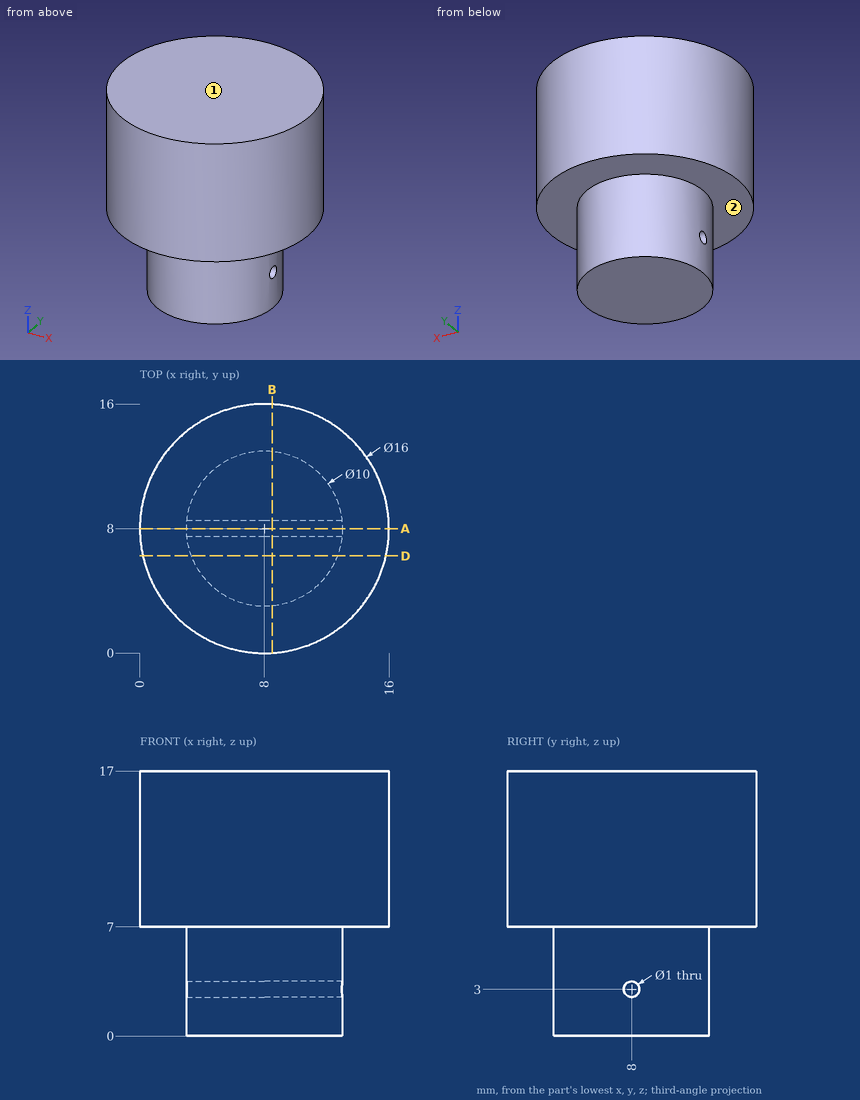
The figure shows three views and two pictorial views of one solid part (mm, origin at its lowest corner). Answer the questions. A direction names the side the tool comes from. Round coordinates to 2 decimals unless told otherwise and drop trailing zeros. Write each loop counter-clockwise with the first axis right and the second up, starting at its lowest first coordinate (ties: lowest second). Pieces come first, ordered by that corner, then holes. Notation, with made-up numbers: M 29,26 L 85,26 A20 ccw 85,60 Z; hole C 5.25,-24.5 d2. An arc over 180 degrees is marked long. Write each question's results on one line, items separated by ' | '. Start each with the question number.
(1) The part is cut by section B-B, the plane x = 8.5. Write down the section's boundary in (y, z), and give its area (3 significant figures).
(2) Find the intervals of material crossed by line 1 (Z direction, x = 6.55, y = 8); line 2 (Z direction, x = 10.75, y = 12.25); line 3 (X direction, y = 10.25, z = 11), in increasing order.
(3) The part is cut by section D-D, the plane y = 6.25. Write down the section's boundary in (x, z).
(4) For the marked faces 1 and 2, determine the directions among +Z, -Z, +X, -X, +Y, -Y from which every point of the face is accessible in a straight line to the end or side of a thin tool.
(5) The part is cut by section A-A, the plane y = 8. Write down the section's boundary in (x, z), and give its area (3 significant figures).
(6) Each of these flat-tipped pins is pushed along its axis until it touches: P1, Ø1.5, axis at x = 7, y = 2, coming from the -Z side; P2, Ø1.5, axis at y = 2.5, z = 7.5, coming from the -X side; P3, Ø2, axis at x = 13, z = 13.5, coming from the +Y side. Where does it stop, or does it pass through?
Worked answers:
1) outline: M 0.02,7 L 3.03,7 L 3.03,0 L 12.97,0 L 12.97,7 L 15.98,7 L 15.98,17 L 0.02,17 Z; hole C 8,3 d1 | area: 229 mm²
2) line 1: z = 0 to 2.5, 3.5 to 17 | line 2: z = 7 to 17 | line 3: x = 0.32 to 15.68
3) outline: M 0.19,7 L 3.32,7 L 3.32,0 L 12.68,0 L 12.68,7 L 15.81,7 L 15.81,17 L 0.19,17 Z
4) face 1: +Z, +X, -X, +Y, -Y | face 2: -Z
5) outline: M 0,7 L 3,7 L 3,3.5 L 13,3.5 L 13,7 L 16,7 L 16,17 L 0,17 Z; M 3,0 L 13,0 L 13,2.5 L 3,2.5 Z | area: 220 mm²
6) P1: stops at z = 7 | P2: stops at x = 1.56 | P3: stops at y = 14.93
